For this review, take the finished solid that the model builds, in its own axes (mm). Face numbers are marked on the shaded views. A direction names the side the tool comes from. Give positions to 0.01 mm unless a question says otherwise; leave off trailing zeros. Order: outer loops, then holes, each group sorted by start corner. A loop starts at its lowest first (then second) coordinate and runs counter-clockwise, first axis right, second up. Notation, with made-up numbers: (27, 1.5) - (79, 1.5) arc R11 ccw to (79, 16.5) - close; hole circle Ø6 at (75.25, 79). An arc over 180 degrees is marked (long way). Use a Markdown table: item, result. Add a question column.
1) Machinability: for the marked faces 4 and 5, which of the approach directions +Z, -Z, +X, -X, +Y, -Y give a long, thin tool a straight path to every point of the face, cutting with its end or side? Answer none if there is none.
2) Wall thickness on L1, parallel to Z at x = 2.5, y = -0.5; L2, parallel to Y at x = -2.5, z = 1.15; L3, parallel to X at y = -3.25, z = -0.1: over which ranges is each line inside the solid? List them lowest first.
3) We need section B-B on z = 0.7. Write out the cut boundary in (x, y), then the cut area to 3 significant figures.
4) We need section A-A on y = 0. Write out the cut boundary in (x, z).
5) Clearance check with flat-ended pins moving along their axes: P1, Ø2.5, axis at x = 1, y = -0.5, coming from the +Z side; P2, Ø1.5, axis at x = 0, y = 0, coming from the -Z side; P3, Ø0.8, axis at y = -3, z = 0.5, coming from the +X side. State where each tip first meets the part, or that it passes through.
6) We need section D-D on y = 2.25. Write out the cut boundary in (x, z), then the cut area to 3 significant figures.
7) Mouldability with a two-part tool opening along Y and no side actions: class the marked faces 1, 2 and 3 as released by +Y, released by -Y, zero draft, split by the parting line, or undercut.
8) We need section C-C on x = -0.75. Write out the cut boundary in (y, z), then the cut area to 3 significant figures.
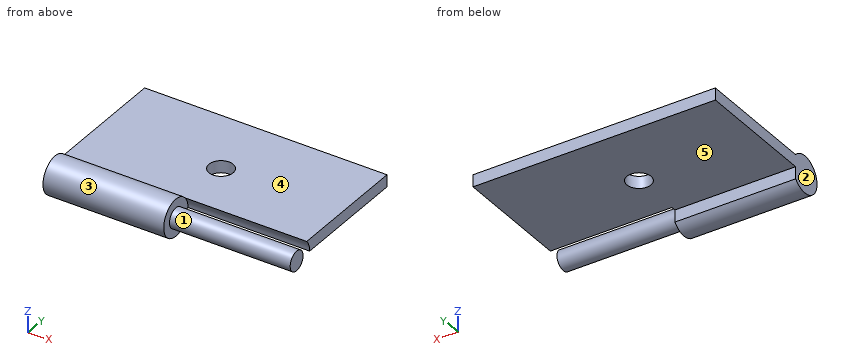
```python
from build123d import *

# Parameters (mm, degrees)
F0_W      = 10.0359702483
F0_H      = 5.6423433125
F1_DEPTH  = 1
F2_R      = 0.7668699523
F3_DEPTH  = 10.08
F4_DEPTH  = 5
F5_R      = 0.4064089658
F6_DEPTH  = 10
F8_D      = 1
F8_DEPTH  = 2
F8_TIP    = 0.3004303095
F9_W      = 5.0608886507
F9_H      = 0.5
F10_DEPTH = 25


with BuildPart() as f1:
    # F0 (on Top) → F1 (new body)
    with BuildSketch(Plane.XY):
        Rectangle(F0_W, F0_H)
    extrude(amount=F1_DEPTH)

    # F2 (on face) → F3 (cut)
    with BuildSketch(Plane(origin=(-5.0179851241, 0, 0), x_dir=(0, -1, 0), z_dir=(-1, 0, 0))):
        with Locations((2.8211716563, 0.5)):
            Circle(F2_R)
    extrude(amount=-F3_DEPTH, mode=Mode.SUBTRACT)

    # F2 (on face) → F4 (join)
    with BuildSketch(Plane(origin=(-5.0179851241, 0, 0), x_dir=(0, -1, 0), z_dir=(-1, 0, 0))):
        with Locations((2.8211716563, 0.5)):
            Circle(F2_R)
    extrude(amount=-F4_DEPTH)

    # F5 (on face) → F6 (join)
    with BuildSketch(Plane(origin=(-5.0179851241, 0, 0), x_dir=(0, -1, 0), z_dir=(-1, 0, 0))):
        with Locations((2.8211716563, 0.5)):
            Circle(F5_R)
    extrude(amount=-F6_DEPTH)

    # F8
    with Locations(Plane.XY.offset(1)):
        with Locations((0, 0)):
            Hole(F8_D / 2, depth=F8_DEPTH)
            with Locations((0, 0, -(F8_DEPTH + F8_TIP / 2))):  # 118° drill point
                Cone(0, F8_D / 2, F8_TIP, mode=Mode.SUBTRACT)

    # F9 (on face) → F10 (cut)
    with BuildSketch(Plane.YZ.offset(5.0179851241)):
        with Locations((0.2907273309, 0.25)):
            Rectangle(F9_W, F9_H)
    extrude(amount=-F10_DEPTH, mode=Mode.SUBTRACT)


solid = f1.part
```
Checked values:
| question | item | result |
|---|---|---|
| 1 | face 4 | +Z, +X, -X, +Y |
| 1 | face 5 | -Z, +X, -X, +Y |
| 2 | L1 | 0.5 to 1 |
| 2 | L2 | -3.23 to -2.41 |
| 2 | L3 | -5.02 to -0.02 |
| 3 | outline | (-5.02, -3.56) - (-0.02, -3.56) - (-0.02, -3.17) - (4.98, -3.17) - (4.98, -2.47) - (-0.02, -2.47) - (-0.02, -2.08) - (5.02, -2.08) - (5.02, 2.82) - (-5.02, 2.82) - close; hole circle Ø1 at (0, 0) |
| 3 | area | 59.4 mm² |
| 4 | outline | (-5.02, 0.5) - (-0.5, 0.5) - (-0.5, 1) - (-5.02, 1) - close; (0.5, 0.5) - (5.02, 0.5) - (5.02, 1) - (0.5, 1) - close |
| 5 | P1 | z = 1 |
| 5 | P2 | z = 0.5 |
| 5 | P3 | x = 4.98 |
| 6 | outline | (-5.02, 0.5) - (5.02, 0.5) - (5.02, 1) - (-5.02, 1) - close |
| 6 | area | 5.02 mm² |
| 7 | face 1 | undercut |
| 7 | face 2 | zero draft |
| 7 | face 3 | split by the parting line |
| 8 | outline | (-2.24, 0) - (-2.24, 0.5) - (2.82, 0.5) - (2.82, 1) - (-2.24, 1) arc R0.77 ccw (long way) to start |
| 8 | area | 4.25 mm² |
